Check sheet for the modelled part. Datum: model origin and axes. Units: mm. A direction names the side the tool comes from. Round coordinates to 2 decimals unless told otherwise and drop trailing zeros. Write each loop counter-clockwise with the first axis right and the second up, starting at its lowest first coordinate (ties: lowest second). Pieces come first, ordered by that corner, then holes. Notation, with made-up numbers: M 83,13 L 138,13 A20 cw 138,23 Z; hole C 40,-37 d6. An arc over 180 degrees is marked long. Put each result on its own line as item: value.
```python
from build123d import *

# Parameters (mm, degrees)
EXTRUDE_THIN1_DEPTH         = 50
BOSS_EXTRUDE1_DEPTH         = 5
EXTRUDE_THIN3_DEPTH         = 5
EXTRUDE_THIN3_DEPTH_BACK    = 5
RIB6_REACH                  = 122.433
SKETCH4_WALL_W              = 296.6238277
SKETCH4_WALL_H              = 10
SKETCH5_W                   = 50
SKETCH5_H                   = 40
BOSS_EXTRUDE2_DEPTH         = 10
FILLET1_RADIUS              = 20
FILLET1_LENGTH              = 10
SKETCH6_R                   = 8
CUT_EXTRUDE1_DEPTH          = 132.77253128
FILLET2_R                   = 5
FILLET1_OF_MIRROR1_2_RADIUS = 20
FILLET1_OF_MIRROR1_2_LENGTH = 10
FILLET2_OF_MIRROR1_R        = 5


with BuildPart() as part:
    # Sketch1 → Extrude-Thin1 (new body)
    with BuildSketch(Plane.XY):
        with BuildLine():
            ThreePointArc((40, 0), (0, 40), (-40, 0))
            Line((-40, 0), (-30, 0))
            ThreePointArc((-30, 0), (0, 30), (30, 0))
            Line((30, 0), (40, 0))
        make_face()
    extrude(amount=EXTRUDE_THIN1_DEPTH)

    # Sketch2 → Boss-Extrude1 (add)
    with BuildSketch(Plane.XY):
        with BuildLine():
            Line((-30, 0), (-40, 0))
            ThreePointArc((-40, 0), (-39.886965034, 3.004999227), (-39.548498982, 5.993014955))
            Line((-39.548498982, 5.993014955), (-25, 102))
            ThreePointArc((-25, 102), (0, 77), (25, 102))
            Line((25, 102), (39.548498982, 5.993014955))
            ThreePointArc((39.548498982, 5.993014955), (39.886965034, 3.004999227), (40, 0))
            Line((40, 0), (30, 0))
            ThreePointArc((30, 0), (0, 30), (-30, 0))
        make_face()
    extrude(amount=BOSS_EXTRUDE1_DEPTH)

    # Sketch3 → Extrude-Thin3 (add, two sides: drawn at the far end of the back side and taken through both)
    with BuildSketch(Plane.XY.offset(5).offset(-EXTRUDE_THIN3_DEPTH_BACK)):
        with BuildLine():
            ThreePointArc((-25, 102), (0, 77), (25, 102))
            Line((25, 102), (16, 102))
            ThreePointArc((16, 102), (0, 86), (-16, 102))
            Line((-16, 102), (-25, 102))
        make_face()
    extrude(amount=EXTRUDE_THIN3_DEPTH + EXTRUDE_THIN3_DEPTH_BACK)

    # Sketch4 wall → Rib6 (add, up to next)
    with BuildSketch(Plane(origin=(0, 58.5, 29.5), x_dir=(0, -0.688260431919, 0.725463698509), z_dir=(0, -0.725463698509, -0.688260431919)), mode=Mode.PRIVATE) as rib6_sk1:
        Rectangle(SKETCH4_WALL_W, SKETCH4_WALL_H)
    rib6_tool1 = extrude(rib6_sk1.sketch, amount=RIB6_REACH, mode=Mode.PRIVATE) - part.part
    add(rib6_tool1.solids().sort_by_distance((0, 58.5, 29.5))[0])

    # Sketch5 → Boss-Extrude2 (add)
    with BuildSketch(Plane(origin=(0, 0, 0), x_dir=(1, 0, 0), z_dir=(0, 1, 0))):
        with Locations((55, -25)):
            Rectangle(SKETCH5_W, SKETCH5_H)
    boss_extrude2 = extrude(amount=BOSS_EXTRUDE2_DEPTH)

    # Fillet1: full round fillet: the end face becomes a half cylinder, R = half its width
    fillet1_face = Plane((80, 5, 25), x_dir=(0, 1, 0), z_dir=(1, 0, 0))  # on the end face: x along it, z out of the body
    fillet1_slab = fillet1_face.offset(-FILLET1_RADIUS / 2) * Box(FILLET1_LENGTH, 2 * FILLET1_RADIUS, FILLET1_RADIUS, mode=Mode.PRIVATE)  # the body's end, R deep
    fillet1_round = Plane((60, 5, 25), x_dir=(1, 0, 0), z_dir=(0, 1, 0)) * Cylinder(FILLET1_RADIUS, FILLET1_LENGTH, mode=Mode.PRIVATE)  # its axis R under the face
    add(fillet1_slab - fillet1_round, mode=Mode.SUBTRACT)

    # Sketch6 → Cut-Extrude1 (cut, through all)
    with BuildSketch(Plane(origin=(0, 10, 0), x_dir=(1, 0, 0), z_dir=(0, 1, 0))):
        with Locations(Location((60, -25, 0), (0, 0, 270))):
            Circle(SKETCH6_R)
    cut_extrude1 = extrude(amount=-CUT_EXTRUDE1_DEPTH, mode=Mode.SUBTRACT)

    # Fillet2
    fillet2_edges = [part.edges().sort_by_distance(p)[0] for p in [
        (39.244898063, 7.996507478, 5),
        (39.886965034, 3.004999227, 5),
        (39.681187851, 5.040171699, 45),
    ]]
    fillet(fillet2_edges, radius=FILLET2_R - 0.0001)  # a hair under: the kernel refuses the full size

    # Mirror1: Boss-Extrude2, Cut-Extrude1 across plane
    add(boss_extrude2.mirror(Plane(origin=(0, 0, 0), x_dir=(0, 0, 1), z_dir=(1, 0, 0))))
    add(cut_extrude1.mirror(Plane(origin=(0, 0, 0), x_dir=(0, 0, 1), z_dir=(1, 0, 0))), mode=Mode.SUBTRACT)

    # Fillet1 of Mirror1 2: full round fillet: the end face becomes a half cylinder, R = half its width
    fillet1_of_mirror1_2_face = Plane((-80, 5, 25), x_dir=(0, 1, 0), z_dir=(-1, 0, 0))  # on the end face: x along it, z out of the body
    fillet1_of_mirror1_2_slab = fillet1_of_mirror1_2_face.offset(-FILLET1_OF_MIRROR1_2_RADIUS / 2) * Box(FILLET1_OF_MIRROR1_2_LENGTH, 2 * FILLET1_OF_MIRROR1_2_RADIUS, FILLET1_OF_MIRROR1_2_RADIUS, mode=Mode.PRIVATE)  # the body's end, R deep
    fillet1_of_mirror1_2_round = Plane((-60, 5, 25), x_dir=(-1, 0, 0), z_dir=(0, 1, 0)) * Cylinder(FILLET1_OF_MIRROR1_2_RADIUS, FILLET1_OF_MIRROR1_2_LENGTH, mode=Mode.PRIVATE)  # its axis R under the face
    add(fillet1_of_mirror1_2_slab - fillet1_of_mirror1_2_round, mode=Mode.SUBTRACT)

    # Fillet2 of Mirror1
    fillet2_of_mirror1_edges = [part.edges().sort_by_distance(p)[0] for p in [
        (-39.244898063, 7.996507478, 5),
        (-39.886965034, 3.004999227, 5),
        (-39.681187851, 5.040171699, 45),
    ]]
    fillet(fillet2_of_mirror1_edges, radius=FILLET2_OF_MIRROR1_R - 0.0001)  # a hair under: the kernel refuses the full size


solid = part.part
```
1. Scan lines: probe 1 along X at (y, z) = (3, 25); probe 2 along Z at (x, y) = (-60, 3); probe 3 along X at (y, z) = (4.5, 25). Record each from-to range of solid material in increasing order.
Computed values:
probe 1: x = -80 to -68, -52 to -29.85, 29.85 to 52, 68 to 80
probe 2: z = 5 to 17, 33 to 45
probe 3: x = -80 to -68, -52 to -29.66, 29.66 to 52, 68 to 80
2. Cross-section at B-B (y = 26.5). Enter the section's corners in (x, z).
Computed values:
outline: M -36.44,0 L -14.06,0 L -14.06,50 L -29.96,50 L -29.96,5 L -36.44,5 Z; M 14.06,0 L 36.44,0 L 36.44,5 L 29.96,5 L 29.96,50 L 14.06,50 Z
3. Cross-section at C-C (z = 23). Enter the section's corners in (x, y).
Computed values:
outline: M -79.9,0 L -67.75,0 L -67.75,10 L -79.9,10 Z; M -52.25,0 L -30,0 A30 cw 30,0 L 52.25,0 L 52.25,10 L 38.73,10 A40 ccw 5,39.69 L 5,64.67 L -5,64.67 L -5,39.69 A40 ccw -38.73,10 L -52.25,10 Z; M 67.75,0 L 79.9,0 L 79.9,10 L 67.75,10 Z
4. Depth check by flat-ended pin: pin 1 Ø2 at (y, z) = (33.5, 9) entering from +X; pin 2 Ø1.5 at (x, z) = (14.5, 9.5) entering from -Y; pin 3 Ø5 at (x, y) = (49, 3) entering from +Z. Enter the tip coordinate at first touch or a pass-through.
Computed values:
pin 1: stops at x = 23.32
pin 2: stops at y = 25.83
pin 3: stops at z = 45
5. Access from +Z, -Z, +X, -X, +Y, -Y to the whole of each face (thin tool, end or side, straight path). Record for faces 5 (the flat face through (-52, 5, 45)), 6 (the flat face through (-52, 5, 5)), 7 (the flat face through (52, 5, 45)).
Computed values:
face 5: +Z, -X, +Y, -Y
face 6: -Z, -X, +Y, -Y
face 7: +Z, +X, +Y, -Y
6. Release check for a two-part mould opening along Z. For faces 1 (the flat face through (49, 0, 25)), 2 (the cylindrical face through (67.932, 5.07, 23.959)), 3 (the flat face through (-0.07, 58.86, 29.12)), 4 (the cylindrical face through (-67.932, 5.07, 23.959)) record: +Z half, -Z half, draft (parallel to the pull), parting line (faces both ways), or undercut.
Computed values:
face 1: draft
face 2: undercut
face 3: +Z half
face 4: undercut
7. Cross-section at A-A (x = 58). Enter the section's corners in (y, z), then the cut area to 3 significant figures.
Computed values:
outline: M 0,5 L 10,5 L 10,17.25 L 0,17.25 Z; M 0,32.75 L 10,32.75 L 10,45 L 0,45 Z
area: 245 mm2
8. Cross-section at D-D (z = 7). Enter the section's corners in (x, y), then the cut area to 3 significant figures.
Computed values:
outline: M -68.72,0 L -30,0 A30 cw 30,0 L 68.72,0 L 68.72,10 L 38.73,10 A40 ccw 5,39.69 L 5,77.51 A25 ccw 25,102 L 16,102 A16 cw -16,102 L -25,102 A25 ccw -5,77.51 L -5,39.69 A40 ccw -38.73,10 L -68.72,10 Z
area: 2,630 mm2
